Solid Edge part; units mm, degrees
sketch "Sketch1" plane through (0, 0, 0) normal (0, 0, 1) x (1, 0, 0)
  circle A0 centre (29.0561, 24.5311) radius 3.1
  line L0 (-30.1036, 67.91) -> (-30.1036, 57.91)
  line L1 (-30.1036, 57.91) -> (49.8964, 57.91)
  line L2 (49.8964, 57.91) -> (49.8964, 67.91)
  line L3 (49.8964, 67.91) -> (-30.1036, 67.91)
  line L4 (-11.2618, -42.5938) -> (-11.2618, -52.5938)
  line L5 (-11.2618, -52.5938) -> (48.7382, -52.5938)
  line L6 (48.7382, -52.5938) -> (48.7382, -42.5938)
  line L7 (48.7382, -42.5938) -> (-11.2618, -42.5938)
  line L8 (-30.6062, -17.1946) -> (-30.6062, -27.1946)
  line L9 (-30.6062, -27.1946) -> (9.3938, -27.1946)
  line L10 (9.3938, -27.1946) -> (9.3938, -17.1946)
  line L11 (9.3938, -17.1946) -> (-30.6062, -17.1946)
  line L12 (-30.1063, 44.8695) -> (-30.1063, 34.8695)
  line L13 (-30.1063, 34.8695) -> (9.8937, 34.8695)
  line L14 (9.8937, 34.8695) -> (9.8937, 44.8695)
  line L15 (9.8937, 44.8695) -> (-30.1063, 44.8695)
  line L16 (-67.1407, 16.0467) -> (-67.1407, 6.0467)
  line L17 (-67.1407, 6.0467) -> (-37.1407, 6.0467)
  line L18 (-37.1407, 6.0467) -> (-37.1407, 16.0467)
  line L19 (-37.1407, 16.0467) -> (-67.1407, 16.0467)
  circle A1 centre (37.2864, -60.1352) radius 2.9
  circle A2 centre (-19.396, 5.3255) radius 3.1
  line L20 (93.6805, -89.8125) -> (-80.713, -89.8125)
  line L21 (-80.713, -89.8125) -> (-80.713, 73.9073)
  line L22 (-80.713, 73.9073) -> (93.6805, 73.9073)
  line L23 (93.6805, 73.9073) -> (93.6805, -89.8125)
  circle A3 centre (29.0561, -16.0575) radius 3.1
  circle A4 centre (63.9812, -11.3592) radius 3.6
  circle A5 centre (63.9812, 30.6072) radius 3.6
  circle A6 centre (28.9096, 33.5121) radius 2.6
  circle A7 centre (28.9096, -7.7928) radius 2.55
  circle A8 centre (-19.396, 15.5257) radius 2.55
  circle A9 centre (52.9623, -47.5938) radius 1.75
  circle A10 centre (14.8937, -22.1946) radius 1.75
  circle A11 centre (-72.1407, 11.0467) radius 1.75
  circle A12 centre (14.8937, 39.8695) radius 1.75
  circle A13 centre (-35.1036, 62.91) radius 1.75
  circle A14 centre (-35.1063, 39.8695) radius 1.75
  circle A15 centre (-32.1407, 11.0467) radius 1.75
  circle A16 centre (-35.1063, -22.1946) radius 1.75
  circle A17 centre (-15.4173, -47.5938) radius 1.75
  circle A18 centre (54.8964, 62.91) radius 1.75
  circle A19 centre (-0.1136, -79.3352) radius 2.9
  line L24 (34.7864, -77.2352) -> (34.7864, -62.1352)
  line L25 (34.7864, -62.1352) -> (4.4864, -62.1352)
  line L26 (4.4864, -62.1352) -> (4.4864, -77.2352)
  line L27 (4.4864, -77.2352) -> (34.7864, -77.2352)
  circle A20 centre (-0.1136, -60.1352) radius 2.9
  circle A21 centre (37.2864, -79.3352) radius 2.9
extrude "Protrusion1" add sketch "Sketch1" along normal blind 1
sketch "Sketch2" plane through (0, 0, 0) normal (0, 0, 1) x (1, 0, 0)
  line L0 (-67.1407, 6.0467) -> (-37.1407, 6.0467)
  line L1 (-37.1407, 6.0467) -> (-37.1407, 16.0467)
  line L2 (-37.1407, 16.0467) -> (-67.1407, 16.0467)
  line L3 (-67.1407, 16.0467) -> (-67.1407, 6.0467)
  line L4 (-30.1063, 34.8695) -> (9.8937, 34.8695)
  line L5 (9.8937, 34.8695) -> (9.8937, 44.8695)
  line L6 (9.8937, 44.8695) -> (-30.1063, 44.8695)
  line L7 (-30.1063, 44.8695) -> (-30.1063, 34.8695)
  line L8 (-30.6062, -27.1946) -> (9.3938, -27.1946)
  line L9 (9.3938, -27.1946) -> (9.3938, -17.1946)
  line L10 (9.3938, -17.1946) -> (-30.6062, -17.1946)
  line L11 (-30.6062, -17.1946) -> (-30.6062, -27.1946)
  line L12 (-11.2618, -52.5938) -> (48.7382, -52.5938)
  line L13 (48.7382, -52.5938) -> (48.7382, -42.5938)
  line L14 (48.7382, -42.5938) -> (-11.2618, -42.5938)
  line L15 (-11.2618, -42.5938) -> (-11.2618, -52.5938)
  line L16 (-30.1036, 57.91) -> (49.8964, 57.91)
  line L17 (49.8964, 57.91) -> (49.8964, 67.91)
  line L18 (49.8964, 67.91) -> (-30.1036, 67.91)
  line L19 (-30.1036, 67.91) -> (-30.1036, 57.91)
  circle A0 centre (-19.396, 5.3255) radius 3.1
  circle A1 centre (-0.1136, -79.3352) radius 2.9
  circle A2 centre (29.0561, -16.0575) radius 3.1
  circle A3 centre (29.0561, 24.5311) radius 3.1
  line L20 (-80.713, -89.8125) -> (-80.713, 73.9073)
  line L21 (-80.713, 73.9073) -> (93.6805, 73.9073)
  line L22 (93.6805, 73.9073) -> (93.6805, -89.8125)
  line L23 (93.6805, -89.8125) -> (-80.713, -89.8125)
  circle A4 centre (63.9812, -11.3592) radius 20
  circle A5 centre (63.8842, 30.3922) radius 20
  circle A6 centre (28.9096, -7.7928) radius 2.55
  circle A7 centre (-19.396, 15.5257) radius 2.55
  circle A8 centre (28.9096, 33.5121) radius 2.6
  circle A9 centre (-35.1063, -22.1946) radius 1.75
  circle A10 centre (52.9623, -47.5938) radius 1.75
  circle A11 centre (-72.1407, 11.0467) radius 1.75
  circle A12 centre (-35.1036, 62.91) radius 1.75
  circle A13 centre (54.8964, 62.91) radius 1.75
  circle A14 centre (-35.1063, 39.8695) radius 1.75
  circle A15 centre (14.8937, 39.8695) radius 1.75
  circle A16 centre (14.8937, -22.1946) radius 1.75
  circle A17 centre (-15.4173, -47.5938) radius 1.75
  circle A18 centre (-32.1407, 11.0467) radius 1.75
  circle A19 centre (37.2864, -60.1352) radius 2.9
  line L24 (34.7864, -77.2352) -> (34.7864, -62.1352)
  line L25 (34.7864, -62.1352) -> (4.4864, -62.1352)
  line L26 (4.4864, -62.1352) -> (4.4864, -77.2352)
  line L27 (4.4864, -77.2352) -> (34.7864, -77.2352)
  circle A20 centre (37.2864, -79.3352) radius 2.9
  circle A21 centre (-0.1136, -60.1352) radius 2.9
extrude "ExtrudedProtrusion_2" add sketch "Sketch2" against normal blind 1
fillet "Round_2" radius 5 4 edges at (93.6805, 73.9073, 0) (93.6805, -89.8125, 0) (-80.713, 73.9073, 0) (-80.713, -89.8125, 0)
sketch "Sketch3" plane through (0, 0, 0) normal (0, 0, 1) x (1, 0, 0)
  circle A0 centre (28.9096, 33.5121) radius 2.95
  circle A1 centre (28.9096, 33.5121) radius 4
  circle A2 centre (-19.396, 15.5257) radius 2.95
  circle A3 centre (-19.396, 15.5257) radius 4
  circle A4 centre (28.9096, -7.7928) radius 2.95
  circle A5 centre (28.9096, -7.7928) radius 4
extrude "ExtrudedProtrusion_4" add sketch "Sketch3" along normal blind 4
sketch "Sketch4" plane through (0, 0, 0) normal (0, 0, 1) x (1, 0, 0)
  circle A0 centre (63.9812, -11.3592) radius 3.6
  circle A1 centre (63.9812, -11.3592) radius 20
  circle A2 centre (63.9812, 30.6072) radius 3.6
  circle A3 centre (63.8842, 30.3922) radius 20
extrude "Protrusion2" add sketch "Sketch4" against normal up to vertex (1 mm away)
sketch "Sketch5" plane through (0, 0, 0) normal (0, 0, 1) x (1, 0, 0)
  circle A0 centre (37.2864, -60.1352) radius 2.9
  circle A1 centre (37.2864, -79.3352) radius 2.9
  circle A2 centre (-0.1136, -79.3352) radius 2.9
  circle A3 centre (-0.1136, -60.1352) radius 2.9
extrude "ExtrudedProtrusion_7" add sketch "Sketch5" along normal blind 1
sketch "Sketch6" plane through (0, 0, 0) normal (0, 0, 1) x (1, 0, 0)
  circle A0 centre (-0.1136, -60.1352) radius 1.45
  circle A1 centre (-0.1136, -60.1352) radius 2.9
  circle A2 centre (-0.1136, -79.3352) radius 1.45
  circle A3 centre (-0.1136, -79.3352) radius 2.9
  circle A4 centre (37.2864, -79.3352) radius 1.45
  circle A5 centre (37.2864, -79.3352) radius 2.9
  circle A6 centre (37.2864, -60.1352) radius 1.45
  circle A7 centre (37.2864, -60.1352) radius 2.9
extrude "ExtrudedProtrusion_8" add sketch "Sketch6" along normal blind 6
Can you work these out from the model? Positions are in its coordinate system, mm. A direction names the side the tool comes from. Give positions to 0.01 mm unless a question says otherwise; leave off trailing zeros. Loops run counter-clockwise (first coordinate to the right, second up) from the corner with the lowest first, then second, coordinate; pieces in that order, holes last. Notation, with made-up numbers: (14, -30.5) -> (35, -30.5) arc R16 ccw to (35, -0.5) -> close; hole circle Ø8 at (79, 9.5). An arc over 180 degrees is marked (long way). Return JSON: item names as keys, results as strings.
Q1. We'd pull the mould along X, two halves only. Please class faces 1 (the face through (65.642, -8.165, -0.014)), 2 (the face through (27, 31, 4)), 3 (the face through (92.177, -88.387, 0.014)), 4 (the face through (40.05, -61.01, 3.46)): released by +X, released by -X, zero draft, split by the parting line, or undercut.
Checks:
{"face 1": "undercut", "face 2": "zero draft", "face 3": "released by +X", "face 4": "undercut"}
Q2. On a 3-axis mill with a long thin cutter (end or side, diameter ignored), from which of +Z, -Z, +X, -X, +Y, -Y can I reach the whole of each face in a straight line? I mean faces 5 (the face through (28.3, 36.4, 2.5)), 6 (the face through (67.3, 32, 0)), 7 (the face through (-0.49, -63.01, -0.51)). Say none if no direction works.
Checks:
{"face 5": "+Z", "face 6": "+Z, -Z", "face 7": "-Z"}
Q3. For pin 1 Ø10 at (x, y) = (73, -2.5) entering from +Z; pin 2 Ø5 at (x, y) = (37.29, -79.34) entering from -Z; pin 3 Ø2.5 at (x, y) = (29.5, 33.5) entering from +Z; pin 4 Ø1.5 at (y, z) = (19.5, 2) entering from +X, each with a flat end and sliding along its axis, tell me the tip position at first contact or that it passes through.
Checks:
{"pin 1": "stops at z = 1", "pin 2": "stops at z = 0", "pin 3": "passes through", "pin 4": "stops at x = -17.03"}
Q4. I need wall thicknesses on probe 1 along X at (y, z) = (-22.5, 0.25); probe 2 along X at (y, z) = (-10, 0.25); probe 3 along Z at (x, y) = (10.5, -80.5). Which ranges of each line are inside material? Lowest first, please.
Checks:
{"probe 1": "x = -80.71 to -36.83, -33.38 to -30.61, 9.39 to 13.17, 16.62 to 93.68", "probe 2": "x = -80.71 to 27.63, 30.19 to 60.65, 67.31 to 93.68", "probe 3": "z = -1 to 1"}
Q5. I want a section at A-A, the plane y = 50. List the corners of the cut face in (x, z) for me, then the cut area to 3 significant figures.
Checks:
{"outline": "(-80.71, -1) -> (93.68, -1) -> (93.68, 1) -> (-80.71, 1) -> close", "area": "349 mm2"}
